Design review of the part built by this model. Coordinates are the model's own, in mm. Face numbers are marked on the shaded views. A direction names the side the tool comes from. Coordinates: 2 decimals unless noted, no trailing zeros. Order: outer loops, then holes, each group sorted by start corner. A loop starts at its lowest first (then second) coordinate and runs counter-clockwise, first axis right, second up. Notation, with made-up numbers: M -25.75,-4 L 28.25,-4 A16 ccw 28.25,12 Z; hole C 8,3 d1. An arc over 180 degrees is marked long. Use CSV: the item, a comma, the result in double quotes.
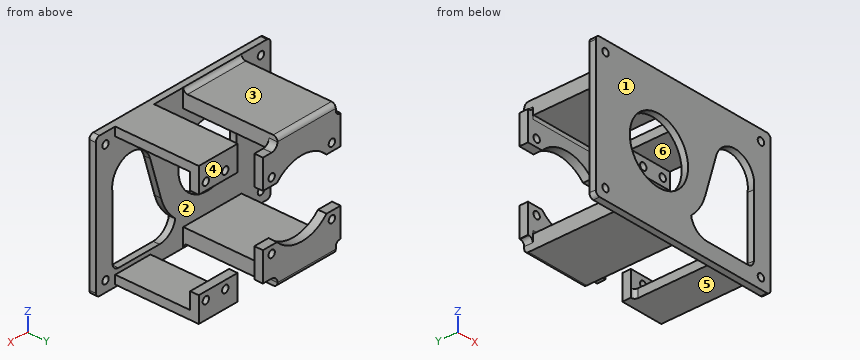
```python
from build123d import *

# Parameters (mm, degrees)
SKETCH_1_R                = 1.65
EXTRUDE_2_DEPTH           = 3
SKETCH_2_W                = 30
SKETCH_2_H                = 5
EXTRUDE_3_DEPTH           = 40
FILLET_1_R                = 2
EXTRUDE_START             = -30
EXTRUDE_4_DEPTH           = 30
EXTRUDE_4_2_OUTLINE_R     = 1.65
EXTRUDE_4_2_DEPTH         = 4
CUT_EXTRUDE_START         = -30
CUT_EXTRUDE_1_DEPTH       = 30
CUT_EXTRUDE_START_2       = -32.5
CUT_EXTRUDE_1_2_DEPTH     = 40
CUT_EXTRUDE_START_3       = -3
CUT_EXTRUDE_1_3_OUTLINE_R = 15
CUT_EXTRUDE_1_3_DEPTH     = 3
SKETCH_7_W                = 18.132065191
SKETCH_7_H                = 4
SKETCH_7_R                = 10
SKETCH_7_W_2              = 20
EXTRUDE_6_DEPTH           = 35
SKETCH_9_W                = 20
SKETCH_9_H                = 11.65
SKETCH_9_R                = 1.65
EXTRUDE_7_DEPTH           = 4
CUT_EXTRUDE_START_4       = -31.5
CUT_EXTRUDE_2_DEPTH       = 4
CUT_EXTRUDE_START_5       = -39
CUT_EXTRUDE_2_2_OUTLINE_R = 10
CUT_EXTRUDE_2_2_DEPTH     = 40
CUT_EXTRUDE_START_6       = -1000
CUT_EXTRUDE_3_DEPTH       = 1000
SKETCH_13_W               = 30
SKETCH_13_H               = 1.5
EXTRUDE_8_DEPTH           = 40


with BuildPart() as part:
    # 草图1 → 凸台-拉伸2 (new body)
    with BuildSketch(Plane(origin=(0, 0, 0), x_dir=(1, 0, 0), z_dir=(0, 1, 0))):
        with BuildLine():
            Line((-43, 32.5), (43, 32.5))
            ThreePointArc((43, 32.5), (44.414213562, 31.914213562), (45, 30.5))
            Line((45, 30.5), (45, -30.5))
            ThreePointArc((45, -30.5), (44.414213562, -31.914213562), (43, -32.5))
            Line((43, -32.5), (-43, -32.5))
            ThreePointArc((-43, -32.5), (-44.414213562, -31.914213562), (-45, -30.5))
            Line((-45, -30.5), (-45, 30.5))
            ThreePointArc((-45, 30.5), (-44.414213562, 31.914213562), (-43, 32.5))
        make_face()
        with Locations(Location((-40, 27.5, 0), (0, 0, 270))):
            Circle(SKETCH_1_R, mode=Mode.SUBTRACT)
        with Locations(Location((40, 27.5, 0), (0, 0, 270))):
            Circle(SKETCH_1_R, mode=Mode.SUBTRACT)
        with Locations(Location((-40, -27.5, 0), (0, 0, 270))):
            Circle(SKETCH_1_R, mode=Mode.SUBTRACT)
        with Locations(Location((40, -27.5, 0), (0, 0, 270))):
            Circle(SKETCH_1_R, mode=Mode.SUBTRACT)
    extrude(amount=EXTRUDE_2_DEPTH)

    # 草图2 → 凸台-拉伸3 (add)
    with BuildSketch(Plane(origin=(0, 3, 0), x_dir=(1, 0, 0), z_dir=(0, 1, 0))):
        with Locations((-15, 28)):
            Rectangle(SKETCH_2_W, SKETCH_2_H)
        with Locations((-15, -28)):
            Rectangle(SKETCH_2_W, SKETCH_2_H)
    extrude(amount=EXTRUDE_3_DEPTH)

    # 圆角1
    fillet_1_edges = [part.edges().sort_by_distance(p)[0] for p in [
        (-15, 3, -30.5),
    ]]
    fillet(fillet_1_edges, radius=FILLET_1_R - 0.0001)  # a hair under: the kernel refuses the full size

    # 凸台-拉伸4: read off the stored shape, not the designer's step
    # 凸台-拉伸4 outline → 凸台-拉伸4 (add)
    with BuildSketch(Plane.YZ.offset(EXTRUDE_START)):
        with BuildLine():
            ThreePointArc((5, 30.5), (3.585786438, 31.085786438), (3, 32.5))
            Line((3, 32.5), (3, 30.5))
            Line((3, 30.5), (5, 30.5))
        make_face()
    extrude(amount=EXTRUDE_4_DEPTH)

    # Extrude 4 2 outline → Extrude 4 2 (add)
    # profile 1 of 2: a face of its own
    with BuildSketch(Plane(origin=(0, 43, 0), x_dir=(1, 0, 0), z_dir=(0, 1, 0))):
        with BuildLine():
            Line((7.5, 12), (7.5, 25.5))
            Line((7.5, 25.5), (3, 25.5))
            ThreePointArc((3, 25.5), (0.878679656, 26.378679656), (0, 28.5))
            Line((0, 28.5), (0, 30.5))
            Line((0, 30.5), (-30, 30.5))
            Line((-30, 30.5), (-30, 27.5))
            ThreePointArc((-30, 27.5), (-30.585786438, 26.085786438), (-32, 25.5))
            Line((-32, 25.5), (-32.5, 25.5))
            Line((-32.5, 25.5), (-32.5, 12))
            Line((-32.5, 12), (-25.237739203, 12))
            ThreePointArc((-25.237739203, 12), (-12.5, 17.5), (0.237739203, 12))
            Line((0.237739203, 12), (7.5, 12))
        make_face()
        with Locations((-28, 15.5)):
            Circle(EXTRUDE_4_2_OUTLINE_R, mode=Mode.SUBTRACT)
        with Locations((3, 15.5)):
            Circle(EXTRUDE_4_2_OUTLINE_R, mode=Mode.SUBTRACT)
    # profile 2 of 2: a face of its own
    with BuildSketch(Plane(origin=(0, 43, 0), x_dir=(1, 0, 0), z_dir=(0, 1, 0))):
        with BuildLine():
            Line((-25.237739203, -12), (-32.5, -12))
            Line((-32.5, -12), (-32.5, -25.5))
            Line((-32.5, -25.5), (-32, -25.5))
            ThreePointArc((-32, -25.5), (-30.585786438, -26.085786438), (-30, -27.5))
            Line((-30, -27.5), (-30, -30.5))
            Line((-30, -30.5), (0, -30.5))
            Line((0, -30.5), (0, -28.5))
            ThreePointArc((0, -28.5), (0.878679656, -26.378679656), (3, -25.5))
            Line((3, -25.5), (7.5, -25.5))
            Line((7.5, -25.5), (7.5, -12))
            Line((7.5, -12), (0.237739203, -12))
            ThreePointArc((0.237739203, -12), (-12.5, -17.5), (-25.237739203, -12))
        make_face()
        with Locations((-28, -15.5)):
            Circle(EXTRUDE_4_2_OUTLINE_R, mode=Mode.SUBTRACT)
        with Locations((3, -15.5)):
            Circle(EXTRUDE_4_2_OUTLINE_R, mode=Mode.SUBTRACT)
    extrude(amount=EXTRUDE_4_2_DEPTH)

    # 切除-拉伸1: read off the stored shape, not the designer's step
    # 切除-拉伸1 outline → 切除-拉伸1 (add)
    with BuildSketch(Plane.YZ.offset(CUT_EXTRUDE_START)):
        with BuildLine():
            ThreePointArc((40, 25.5), (42.121320344, 24.621320344), (43, 22.5))
            Line((43, 22.5), (43, 25.5))
            Line((43, 25.5), (40, 25.5))
        make_face()
        with BuildLine():
            ThreePointArc((43, -22.5), (42.121320344, -24.621320344), (40, -25.5))
            Line((40, -25.5), (43, -25.5))
            Line((43, -25.5), (43, -22.5))
        make_face()
    extrude(amount=CUT_EXTRUDE_1_DEPTH)

    # Cut-Extrude 1 2 outline → Cut-Extrude 1 2 (cut)
    with BuildSketch(Plane.YZ.offset(CUT_EXTRUDE_START_2)):
        with BuildLine():
            Line((47, 30.5), (45, 30.5))
            ThreePointArc((45, 30.5), (46.414213562, 29.914213562), (47, 28.5))
            Line((47, 28.5), (47, 30.5))
        make_face()
        with BuildLine():
            Line((47, -30.5), (47, -28.5))
            ThreePointArc((47, -28.5), (46.414213562, -29.914213562), (45, -30.5))
            Line((45, -30.5), (47, -30.5))
        make_face()
    extrude(amount=CUT_EXTRUDE_1_2_DEPTH, mode=Mode.SUBTRACT)

    # Cut-Extrude 1 3 outline → Cut-Extrude 1 3 (cut)
    with BuildSketch(Plane(origin=(0, 3, 0), x_dir=(1, 0, 0), z_dir=(0, 1, 0)).offset(CUT_EXTRUDE_START_3)):
        with Locations((-12.5, 0)):
            Circle(CUT_EXTRUDE_1_3_OUTLINE_R)
    extrude(amount=CUT_EXTRUDE_1_3_DEPTH, mode=Mode.SUBTRACT)

    # 草图7 → 凸台-拉伸6 (add)
    with BuildSketch(Plane(origin=(0, 3, 0), x_dir=(1, 0, 0), z_dir=(0, 1, 0))):
        with Locations((25.933967405, 29.5)):
            Rectangle(SKETCH_7_W, SKETCH_7_H)
        with Locations(Location((26.586442662, -8.5, 0), (0, 0, 270))):
            Circle(SKETCH_7_R)
        with Locations((25, -30.5)):
            Rectangle(SKETCH_7_W_2, SKETCH_7_H)
    extrude(amount=EXTRUDE_6_DEPTH)

    # 草图9 → 凸台-拉伸7 (add)
    # profile 1 of 2: a face of its own
    with BuildSketch(Plane(origin=(0, 38, 0), x_dir=(1, 0, 0), z_dir=(0, 1, 0))):
        with Locations((25, 25.675)):
            Rectangle(SKETCH_9_W, SKETCH_9_H)
        with Locations(Location((31.355501541, 23.5, 0), (0, 0, 270))):
            Circle(SKETCH_9_R, mode=Mode.SUBTRACT)
        with Locations(Location((21.355501541, 23.5, 0), (0, 0, 270))):
            Circle(SKETCH_9_R, mode=Mode.SUBTRACT)
    # profile 2 of 2: a face of its own
    with BuildSketch(Plane(origin=(0, 38, 0), x_dir=(1, 0, 0), z_dir=(0, 1, 0))):
        with Locations((25, -26.675)):
            Rectangle(SKETCH_9_W, SKETCH_9_H)
        with Locations(Location((31.355501541, -24.5, 0), (0, 0, 270))):
            Circle(SKETCH_9_R, mode=Mode.SUBTRACT)
        with Locations(Location((21.355501541, -24.5, 0), (0, 0, 270))):
            Circle(SKETCH_9_R, mode=Mode.SUBTRACT)
    extrude(amount=EXTRUDE_7_DEPTH)

    # 切除-拉伸2: read off the stored shape, not the designer's step
    # 切除-拉伸2 outline → 切除-拉伸2 (add)
    with BuildSketch(Plane.XY.offset(CUT_EXTRUDE_START_4)):
        with BuildLine():
            ThreePointArc((15.367934809, 38), (16.42859498, 37.560660171), (16.867934809, 36.5))
            Line((16.867934809, 36.5), (16.867934809, 38))
            Line((16.867934809, 38), (15.367934809, 38))
        make_face()
    extrude(amount=CUT_EXTRUDE_2_DEPTH)

    # Cut-Extrude 2 2 outline → Cut-Extrude 2 2 (cut)
    with BuildSketch(Plane(origin=(0, 38, 0), x_dir=(1, 0, 0), z_dir=(0, 1, 0)).offset(CUT_EXTRUDE_START_5)):
        with Locations((26.586442662, -8.5)):
            Circle(CUT_EXTRUDE_2_2_OUTLINE_R)
    extrude(amount=CUT_EXTRUDE_2_2_DEPTH, mode=Mode.SUBTRACT)

    # 草图11 → 切除-拉伸3 (cut)
    with BuildSketch(Plane(origin=(0, 3, 0), x_dir=(1, 0, 0), z_dir=(0, 1, 0)).offset(CUT_EXTRUDE_START_6)):
        with BuildLine():
            Line((36.351968475, -6.347209811), (36.351968475, 22.5))
            ThreePointArc((36.351968475, 22.5), (35.473288819, 24.621320344), (33.351968475, 25.5))
            Line((33.351968475, 25.5), (12.201289858, 25.5))
            ThreePointArc((12.201289858, 25.5), (6.908991343, 23.578301134), (4.082716458, 18.708648131))
            ThreePointArc((4.082716458, 18.708648131), (8.569131741, 13.457031161), (11.447301334, 7.178214179))
            Line((11.447301334, 7.178214179), (17.007522129, -11.371285672))
            ThreePointArc((17.007522129, -11.371285672), (24.072672596, 1.178892501), (36.351968475, -6.347209811))
        make_face()
    extrude(amount=CUT_EXTRUDE_3_DEPTH, mode=Mode.SUBTRACT)

    # 草图13 → 凸台-拉伸8 (add)
    with BuildSketch(Plane(origin=(0, 3, 0), x_dir=(1, 0, 0), z_dir=(0, 1, 0))):
        with Locations((-15, 24.75)):
            Rectangle(SKETCH_13_W, SKETCH_13_H)
        with Locations((-15, -24.75)):
            Rectangle(SKETCH_13_W, SKETCH_13_H)
    extrude(amount=EXTRUDE_8_DEPTH)


solid = part.part
```
(1) Wall thickness on probe 1 along X at (y, z) = (1.2, 27.5); probe 2 along Z at (x, y) = (-28, 45.05); probe 3 along Z at (x, y) = (3, 44.6): over which ranges is each line inside the solid? List them lowest first.
The answers:
probe 1,"x = -45 to -41.65, -38.35 to 38.35, 41.65 to 45"
probe 2,"z = -30.5 to -17.15, -13.85 to -12, 12 to 13.85, 17.15 to 30.5"
probe 3,"z = -25.5 to -17.15, -13.85 to -12, 12 to 13.85, 17.15 to 25.5"
(2) Add section D-D on z = 8.5. State the section outline as (x, y) points, and give its area (3 significant figures).
The answers:
outline,"M -45,0 L -24.86,0 L -24.86,3 L -45,3 Z; M -0.14,0 L 16.15,0 L 16.15,3 L -0.14,3 Z; M 36.59,0 L 45,0 L 45,3 L 36.59,3 Z"
area,"135 mm2"
(3) For the marked faces 4, 5 and 6, list the 3-axis set-ups (+Z, -Z, +X, -X, +Y, -Y) from which the entire face can be reached by the end or side of a thin tool; tool diameter is ignored.
The answers:
face 4,"+Z, -Z, +X, +Y"
face 5,"-Z, +X, -X, +Y"
face 6,"+X"
(4) Add section C-C on z = 0. State the section outline as (x, y) points.
The answers:
outline,"M -45,0 L -27.5,0 L -27.5,3 L -45,3 Z; M 2.5,0 L 13.6,0 L 13.6,3 L 2.5,3 Z; M 36.35,0 L 45,0 L 45,3 L 36.35,3 Z"
(5) The part is to be moulded in two halves that separate along Z. For the marked faces 1, 2 and 3, say which applies: pulls with the +Z half, pulls with the -Z half, needs draft (parallel to the pull), parting line crosses it, or undercut.
The answers:
face 1,"needs draft"
face 2,"undercut"
face 3,"pulls with the +Z half"
(6) Add section B-B on x = 24. State the section outline as (y, z) points.
The answers:
outline,"M 0,-32.5 L 3,-32.5 L 3,-31.5 L 42,-31.5 L 42,-19.85 L 38,-19.85 L 38,-27.5 L 3,-27.5 L 3,-25.5 L 0,-25.5 Z; M 0,18.16 L 3,18.16 L 3,28.5 L 38,28.5 L 38,20.85 L 42,20.85 L 42,32.5 L 0,32.5 Z"
(7) Add section A-A on y = 8.5. State the section outline as (x, z) points.
The answers:
outline,"M -30,-30.5 L 0,-30.5 L 0,-24 L -30,-24 Z; M -30,24 L 0,24 L 0,30.5 L -30,30.5 Z; M 15,28.5 L 35,28.5 L 35,32.5 L 15,32.5 Z; M 16.87,-31.5 L 35,-31.5 L 35,-27.5 L 16.87,-27.5 Z"
(8) Clearance check with flat-ended pins moving along their axes: P1, Ø3, axis at x = -21, y = 25, coming from the +Z side; P2, Ø4, axis at x = -31, y = 14.5, coming from the -Z side; P3, Ø8, axis at x = 33.5, z = 5, coming from the -Y side; P4, Ø13, axis at x = 26, z = -27, coming from the +Y side. State where each tip first meets the part, or that it passes through.
The answers:
P1,"stops at z = 30.5"
P2,"stops at z = -30.5"
P3,"stops at y = 0"
P4,"stops at y = 42"
